Autodesk Inventor part; units mm, degrees
ref_plane "YZ Plane" through (0, 0, 0) normal (1, 0, 0) x (0, 1, 0)
ref_plane "XZ Plane" through (0, 0, 0) normal (0, 1, 0) x (-1, 0, 0)
ref_plane "XY Plane" through (0, 0, 0) normal (0, 0, 1) x (1, 0, 0)
sketch "Эскиз1" plane through (0, 0, 0) normal (0, 1, 0) x (-1, 0, 0)
  line L0 (-16, 16) -> (16, 16)
  line L1 (16, 16) -> (16, -16)
  line L2 (16, -16) -> (-16, -16)
  line L3 (-16, -16) -> (-16, 16)
  line L4 (-16, 16) -> (16, -16) construction
  line L5 (16, 16) -> (-16, -16) construction
  point P0 (0, 0)
  dimension "d0" = 32
  dimension "d1" = 32
extrude "Выдавливание1" add sketch "Эскиз1" along normal blind 3.5
sketch "Эскиз2" plane through (0, 3.5, 0) normal (0, 1, 0) x (1, 0, 0)
  circle A0 centre (0, 8) radius 1.85
  circle A1 centre (-5.6569, 5.6569) radius 1.85
  circle A2 centre (-8, 0) radius 1.85
  circle A3 centre (-5.6569, -5.6569) radius 1.85
  circle A4 centre (0, -8) radius 1.85
  circle A5 centre (5.6569, -5.6569) radius 1.85
  circle A6 centre (8, 0) radius 1.85
  circle A7 centre (5.6569, 5.6569) radius 1.85
  circle A8 centre (0, 0) radius 4
  circle A9 centre (0, 8) radius 1.85
  circle A10 centre (-5.6569, 5.6569) radius 1.85
  circle A11 centre (-8, 0) radius 1.85
  circle A12 centre (-5.6569, -5.6569) radius 1.85
  circle A13 centre (0, -8) radius 1.85
  circle A14 centre (5.6569, -5.6569) radius 1.85
  circle A15 centre (8, 0) radius 1.85
  circle A16 centre (5.6569, 5.6569) radius 1.85
  circle A17 centre (0, 0) radius 4
  circle A18 centre (0, 8) radius 1.85
  circle A19 centre (-5.6569, 5.6569) radius 1.85
  circle A20 centre (-8, 0) radius 1.85
  circle A21 centre (-5.6569, -5.6569) radius 1.85
  circle A22 centre (0, -8) radius 1.85
  circle A23 centre (5.6569, -5.6569) radius 1.85
  circle A24 centre (8, 0) radius 1.85
  circle A25 centre (5.6569, 5.6569) radius 1.85
  circle A26 centre (0, 0) radius 4
  point P0 (0, 0)
  point P1 (0, -16)
  point P2 (0, -16)
  point P3 (0, -16)
extrude "Выдавливание2" cut sketch "Эскиз2" against normal blind 3.5 contours A0 | A2 | A4 | A6
sketch "Эскиз3" plane through (0, 3.5, 0) normal (0, 1, 0) x (1, 0, 0)
  circle A0 centre (0, 0) radius 6.15
  circle A1 centre (-8, 0) radius 1.85
extrude "Выдавливание3" add sketch "Эскиз3" along normal blind 48.5 contours A0
sketch "Эскиз4" plane through (0, 52, 0) normal (0, 1, 0) x (1, 0, 0)
  circle A0 centre (-8, 0) radius 1.85
  circle A1 centre (-8, 0) radius 5
  point P0 (0, 0)
  point P1 (-6.15, 0)
  dimension "d8" = 10
extrude "Выдавливание4" cut sketch "Эскиз4" against normal up to surface (48.5 mm away)
properties part number "000.001.015 - Стойка площадки высокая"
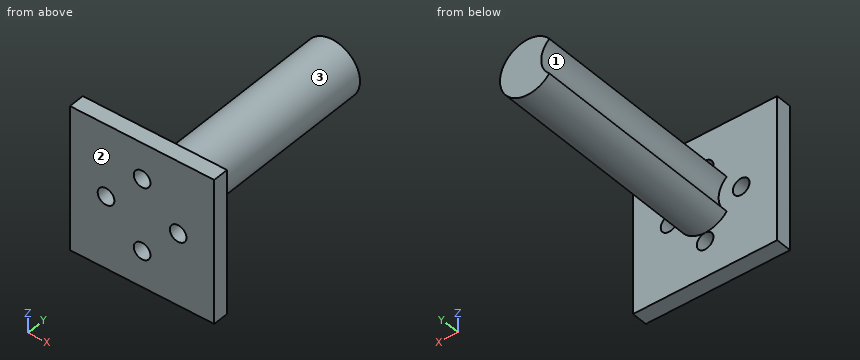
Could you check a few things on this model? Use its own coordinates, in mm. Face numbers are marked on the shaded views. Give positions to 0.01 mm unless a question says otherwise; leave off trailing zeros. Order: outer loops, then holes, each group sorted by start corner. A loop starts at its lowest first (then second) coordinate and runs counter-clockwise, first axis right, second up.
Item 1: If we section it at D-D, the plane y = 28: Write out the boundary of the cut face in (x, z), plus the area to 3 significant figures.
Item 2: If we section it at B-B, the plane x = 8: Write out the boundary of the cut face in (y, z).
Item 3: I'm going to push flat-ended pins straight in: pin 1 (5 mm diameter, centred on x = -8, z = 0, fed in from -Y); pin 2 (3.5 mm diameter, centred on x = 0, z = -8, fed in from -Y); pin 3 (10 mm diameter, centred on y = 33.5, z = 7.5, fed in from +X); pin 4 (10 mm diameter, centred on x = 7.5, y = 18.5, fed in from -Z). Where does each tip first touch, or does it pass through?
Item 4: If we mould it in two halves opening along Z, with no side actions, what happens to the marked faces 1, 2 and 3? For each: pulls with the +Z half, pulls with the -Z half, needs draft (parallel to the pull), parting line crosses it, or undercut.
Item 5: I need wall thicknesses on line 1 (X direction, y = 1.1, z = 0); line 2 (Z direction, x = -8, y = 1.7). Which ranges of each line are inside material? Lowest first, please.
Item 6: If we section it at C-C, the plane z = -1: Write out the boundary of the cut face in (x, y).
Item 7: If we section it at A-A, the plane z = 8: Write out the boundary of the cut face in (x, y).
Values:
1. outline: (-4.8, -3.84) arc R6.15 ccw (long way) to (-4.8, 3.84) arc R5 cw to start
1. area: 102 mm2
2. outline: (0, -16) - (3.5, -16) - (3.5, -1.85) - (0, -1.85) - close; (0, 1.85) - (3.5, 1.85) - (3.5, 16) - (0, 16) - close
3. pin 1: stops at y = 0
3. pin 2: passes through
3. pin 3: stops at x = 5.62
3. pin 4: stops at z = -5.62
4. face 1: undercut
4. face 2: needs draft
4. face 3: parting line crosses it
5. line 1: x = -16 to -9.85, -6.15 to 6.15, 9.85 to 16
5. line 2: z = -16 to -1.85, 1.85 to 16
6. outline: (-16, 0) - (-9.56, 0) - (-9.56, 3.5) - (-16, 3.5) - close; (-6.44, 0) - (6.44, 0) - (6.44, 3.5) - (6.07, 3.5) - (6.07, 52) - (-3.1, 52) - (-3.1, 3.5) - (-6.44, 3.5) - close; (9.56, 0) - (16, 0) - (16, 3.5) - (9.56, 3.5) - close
7. outline: (-16, 0) - (-1.85, 0) - (-1.85, 3.5) - (-16, 3.5) - close; (1.85, 0) - (16, 0) - (16, 3.5) - (1.85, 3.5) - close
